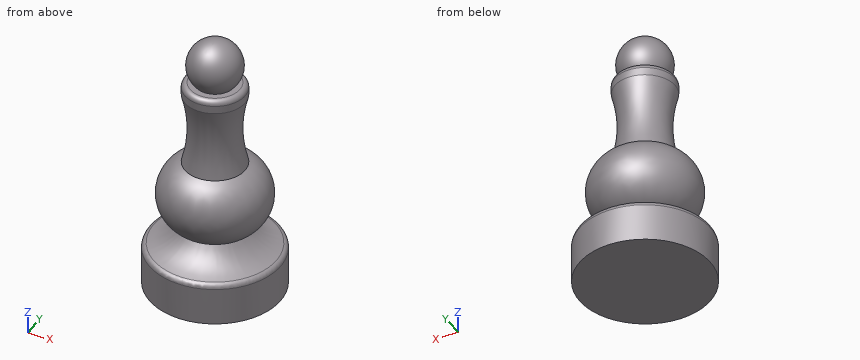
from build123d import *

# Parameters (mm, degrees)
F2_R = 1
F3_R = 1


with BuildPart() as f1:
    # F0 (on Right) → F1 (revolve)
    with BuildSketch(Plane.YZ):
        with BuildLine():
            Line((-12.5, 0), (0, 0))
            Line((0, 0), (0, 50))
            ThreePointArc((0, 50), (-4.609772, 46.936492), (-3.570714, 41.5))
            Line((-3.570714, 41.5), (-5.75, 41.5))
            Line((-5.75, 41.5), (-5.75, 39))
            ThreePointArc((-5.75, 39), (-4.75, 32), (-5.75, 25))
            ThreePointArc((-5.75, 25), (-10.151924, 18.5), (-5.75, 12))
            ThreePointArc((-5.75, 12), (-8.716309, 9.310335), (-12.5, 8))
            Line((-12.5, 8), (-12.5, 0))
        make_face()
    revolve(axis=Axis((0, 0, 25), (0, 0, -1)))

    # F2
    f2_edges = [f1.edges().sort_by_distance(p)[0] for p in [
        (0, 12.5, 8),
    ]]
    fillet(f2_edges, radius=F2_R)

    # F3
    f3_edges = [f1.edges().sort_by_distance(p)[0] for p in [
        (0, 5.75, 41.5),
    ]]
    fillet(f3_edges, radius=F3_R)


solid = f1.part
Geometry: final body of the model. Coordinates: model frame, mm. Coordinates: 2 decimals unless noted, no trailing zeros. Order: outer loops, then holes, each group sorted by start corner. A loop starts at its lowest first (then second) coordinate and runs counter-clockwise, first axis right, second up.
(1) First-contact query: pin 1 (6 mm diameter, centred on x = -4, y = 6.5, fed in from +Z); pin 2 (6 mm diameter, centred on x = 7.5, y = 6, fed in from +Z); pin 3 (5 mm diameter, centred on y = 4, z = 17.5, fed in from -X). Flat tips, straight axial feed; report the tip coordinate or a pass-through.
(2) Section query B-B (z = 34). Return the cut outline in (x, y).
(3) Section query A-A (z = 28). Return the cut outline in (x, y), plus the area to 3 significant figures.
(4) Material intervals for probe 1 along X at (y, z) = (-3.25, 39); probe 2 along Z at (x, y) = (6, -1.75); probe 3 along Z at (x, y) = (6.25, 1.25), sorted ascending.
Solution:
1. pin 1: stops at z = 46.88
1. pin 2: stops at z = 24.59
1. pin 3: stops at x = -10.02
2. outline: circle Ø9.66 at (0, 0)
3. outline: circle Ø10.14 at (0, 0)
3. area: 80.8 mm2
4. probe 1: x = -4.74 to 4.74
4. probe 2: z = 0 to 11.37, 12.22 to 24.78
4. probe 3: z = 0 to 11.23, 12.29 to 24.71
